Autodesk Inventor part; units mm, degrees
ref_plane "YZ Plane" through (0, 0, 0) normal (1, 0, 0) x (0, 1, 0)
ref_plane "XZ Plane" through (0, 0, 0) normal (0, 1, 0) x (-1, 0, 0)
ref_plane "XY Plane" through (0, 0, 0) normal (0, 0, 1) x (1, 0, 0)
sketch "Sketch1" plane through (0, 0, 0) normal (0, 0, 1) x (1, 0, 0)
  line L0 (0, 0) -> (0, 85)
  line L1 (0, 85) -> (160, 85)
  line L2 (160, 85) -> (160, 0)
  line L3 (160, 0) -> (157.6, 0)
  line L4 (157.6, 0) -> (157.6, 82.6)
  line L5 (157.6, 82.6) -> (2.4, 82.6)
  line L6 (2.4, 82.6) -> (2.4, 0)
  line L7 (2.4, 0) -> (0, 0)
  dimension "d0" = 85
  dimension "d1" = 160
  dimension "d2" = 2.4
  dimension "d3" = 82.6
  dimension "d4" = 155.2
extrude "Extrusion1" add sketch "Sketch1" along normal blind 0.9
sketch "Sketch2" plane through (0, 0, 0) normal (-1, 0, 0) x (0, 0, 1)
  line L0 (0, 0) -> (0.9, 0)
  line L1 (0.9, 0) -> (40.9, 0)
  line L2 (0.9, 0) -> (0.9, 85)
  line L3 (0.9, 85) -> (0.9, 0)
  line L4 (40.9, 0) -> (110.9, 0) construction
  line L5 (0.9, 85) -> (0.9, 0)
  line L6 (40.9, 0) -> (0.9, 85)
  dimension "d7" = 40
extrude "Extrusion2" add sketch "Sketch2" against normal blind 2.4
sketch "Sketch3" plane through (160, 0, 0) normal (1, 0, 0) x (0, 0, -1)
  line L0 (-0.9, 0) -> (-0.9, 85)
  line L1 (-0.9, 0) -> (-30.8653, 0)
  line L2 (0, 0) -> (-40.9, 0)
  line L3 (-0.9, 0) -> (-40.9, 0)
  line L4 (0, 85) -> (-0.9, 85)
  line L5 (-0.9, 85) -> (-0.9, 0)
  line L6 (0, 0) -> (-40.9, 0)
  line L7 (-0.9, 85) -> (-40.9, 0)
  line L8 (-0.9, 85) -> (-40.9, 0)
extrude "Extrusion3" add sketch "Sketch3" against normal blind 2.4
sketch "Sketch5" plane through (2.4, 0, 0) normal (1, 0, 0) x (0, 0, -1)
  line L0 (0, 0) -> (-40.9, 0)
  line L1 (-40.9, 0) -> (-0.9, 85)
  line L2 (-0.9, 85) -> (-0.9, 82.6)
  line L3 (-0.9, 85) -> (-0.9, 82.6)
  line L4 (-0.9, 82.6) -> (-39.7706, 0)
  line L5 (-39.7706, 0) -> (-40.9, 0)
extrude "Extrusion5" add sketch "Sketch5" along normal blind 156
sketch "Sketch6" plane through (0, 0, 40.9) normal (0, -1, 0) x (1, 0, 0)
  line L0 (0, -40.9) -> (160, -40.9)
  line L1 (0, 0) -> (0, -40)
  line L2 (0, -40.9) -> (0, 0)
  line L3 (0, 0) -> (160, 0)
  line L4 (0, 0) -> (160, 0)
  line L5 (160, -40.9) -> (160, 0)
  line L6 (160, 0) -> (160, -40.9)
  line L7 (157.6, -40.9) -> (157.6, -1.1294)
  line L8 (160, -40.9) -> (157.6, -40.9)
  line L9 (157.6, -40.9) -> (157.6, -1.1294)
  line L10 (2.4, -1.1294) -> (157.6, -1.1294)
  line L11 (157.6, -1.1294) -> (2.4, -1.1294)
  line L12 (2.4, -1.1294) -> (2.4, -40.9)
  line L13 (2.4, -40.9) -> (0, -40.9)
extrude "Extrusion6" add sketch "Sketch6" along normal blind 12.6 contours L2 L1 L3 L5 L0 L7 L10 L12
properties part number "Front_Chassi"
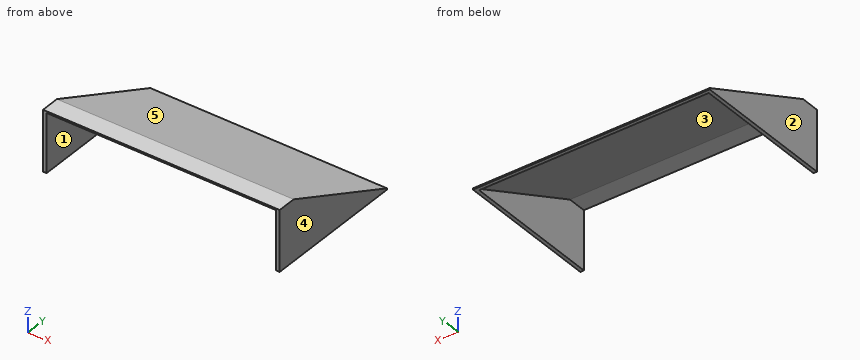
Geometry check sheet. Reference: the model listing, model coordinates, mm. Face numbers are marked on the shaded views. A direction names the side the tool comes from. Coordinates: 2 decimals unless noted, no trailing zeros. Order: outer loops, then holes, each group sorted by start corner. A loop starts at its lowest first (then second) coordinate and runs counter-clockwise, first axis right, second up. Notation, with made-up numbers: (47, 61.5) - (62, 61.5) arc R5 cw to (62, 65.5) - close; hole circle Ø8 at (-17.75, 14). An arc over 180 degrees is marked (long way). Answer in a Markdown table with one row per item. Add a question column.
1) Cross-section at A-A, the plane z = 4.5. Record the cut outline in (x, y), then the cut area to 3 significant figures.
2) Gauge pin test, flat ends, axial feed: P1, Ø3, axis at x = 32.5, y = 38, coming from the +Z side; P2, Ø6, axis at x = 102.5, y = 32.5, coming from the -Z side; P3, Ø5, axis at x = 33, y = 31, coming from the +Z side; P4, Ø3, axis at y = 12, z = 10, coming from the -X side. Record the tip position at first contact, or that the pin passes through.
3) Set-up check for the marked faces 1 and 2: record each of +Z, -Z, +X, -X, +Y, -Y from which the full face is reachable in a straight line by a thin tool's end or side.
4) Material ranges on line 1 along X through (y, z) = (31, 15.5); line 2 along Z through (x, y) = (16.5, 66.5); line 3 along Y through (x, z) = (150, 15), recorded low to high. Write a range as [from, to].
5) Release check for a two-part mould opening along X. For the marked faces 3, 4 and 5 record: +X half, -X half, draft (parallel to the pull), parting line (faces both ways), or undercut.
6) Cross-section at B-B, the plane x = 61. Record the cut outline in (y, z).
Check result:
| question | item | result |
|---|---|---|
| 1 | outline | (0, -12.6) - (2.4, -12.6) - (2.4, 74.95) - (157.6, 74.95) - (157.6, -12.6) - (160, -12.6) - (160, 77.35) - (0, 77.35) - close |
| 1 | area | 804 mm² |
| 2 | P1 | stops at z = 23.72 |
| 2 | P2 | stops at z = 23.06 |
| 2 | P3 | stops at z = 27.49 |
| 2 | P4 | stops at x = 0 |
| 3 | face 1 | -Z, -Y |
| 3 | face 2 | +Z, -Z, -X, +Y, -Y |
| 4 | line 1 | x = [0, 2.4], [157.6, 160] |
| 4 | line 2 | z = [8.48, 9.61] |
| 4 | line 3 | y = [52.64, 55.04] |
| 5 | face 3 | undercut |
| 5 | face 4 | +X half |
| 5 | face 5 | draft |
| 6 | outline | (-12.6, 39.77) - (0, 39.77) - (82.6, 0.9) - (82.6, 0) - (85, 0) - (85, 0.9) - (0, 40.9) - (-12.6, 40.9) - close |
